For this review, take the finished solid that the model builds, in its own axes (mm). Face numbers are marked on the shaded views. A direction names the side the tool comes from. Give positions to 0.01 mm unless a question says otherwise; leave off trailing zeros. Loops run counter-clockwise (first coordinate to the right, second up) from the corner with the lowest first, then second, coordinate; pieces in that order, holes last.
```python
from build123d import *

# Parameters (mm, degrees)
SKETCH1_R           = 6.5
SKETCH1_R_2         = 7.5
BOSS_EXTRUDE1_DEPTH = 15
FILLET2_R           = 1.5
SKETCH4_R           = 3
CUT_EXTRUDE1_DEPTH  = 28


with BuildPart() as part:
    # Sketch1 → Boss-Extrude1 (new body)
    with BuildSketch(Plane.XY):
        with BuildLine():
            Line((-13.5, 0), (-13.5, -24))
            ThreePointArc((-13.5, -24), (-13.060660172, -25.060660172), (-12, -25.5))
            Line((-12, -25.5), (-9.5, -25.5))
            ThreePointArc((-9.5, -25.5), (-8.439339828, -25.939339828), (-8, -27))
            Line((-8, -27), (-8, -175.723012342))
            ThreePointArc((-8, -175.723012342), (0, -197.25), (8, -175.723012342))
            Line((8, -175.723012342), (8, -27))
            ThreePointArc((8, -27), (8.439339828, -25.939339828), (9.5, -25.5))
            Line((9.5, -25.5), (12, -25.5))
            ThreePointArc((12, -25.5), (13.060660172, -25.060660172), (13.5, -24))
            Line((13.5, -24), (13.5, 0))
            ThreePointArc((13.5, 0), (0, 13.5), (-13.5, 0))
        make_face()
        with Locations((0, -185)):
            Circle(SKETCH1_R, mode=Mode.SUBTRACT)
        Circle(SKETCH1_R_2, mode=Mode.SUBTRACT)
    extrude(amount=BOSS_EXTRUDE1_DEPTH)

    # Fillet2
    fillet2_edges = [part.edges().sort_by_distance(p)[0] for p in [
        (-13.060660172, -25.060660172, 15),
        (-10.75, -25.5, 15),
        (-8.439339828, -25.939339828, 15),
        (-8, -101.361506171, 15),
        (8, -101.361506171, 15),
        (8.439339828, -25.939339828, 15),
        (10.75, -25.5, 15),
        (13.060660172, -25.060660172, 15),
        (13.5, -12, 15),
        (0, 13.5, 15),
        (-13.5, -12, 15),
    ]]
    fillet(fillet2_edges, radius=FILLET2_R)

    # Sketch4 → Cut-Extrude1 (cut, through all)
    with BuildSketch(Plane(origin=(13.5, 0, 0), x_dir=(0, 0, -1), z_dir=(1, 0, 0))):
        with Locations((-6.75, -8)):
            Circle(SKETCH4_R)
    extrude(amount=-CUT_EXTRUDE1_DEPTH, mode=Mode.SUBTRACT)


solid = part.part
```
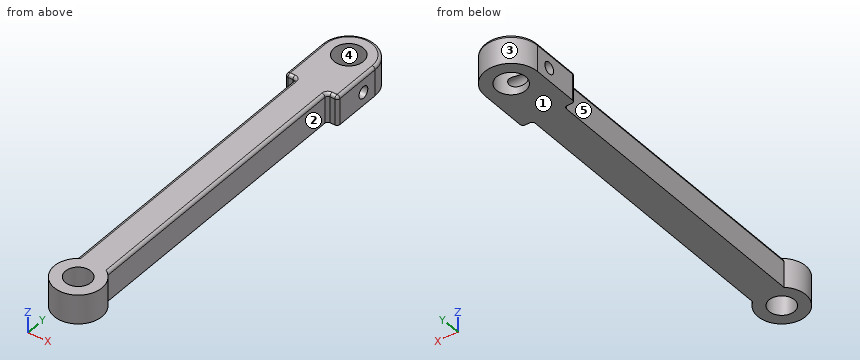
Item 1: Tool access review of the marked faces 4 and 5: name each direction out of +Z, -Z, +X, -X, +Y, -Y from which nothing blocks a thin tool from reaching the whole face with its end or side.
Answer:
face 4: +Z, -Z
face 5: +Z, -Z, -X
Item 2: Take a section at B-B on z = 6.25. Give the boundary of the cut face in (x, y), and give its area (3 significant figures).
Answer:
outline: (-13.5, -24) arc R1.5 ccw to (-12, -25.5) - (-9.5, -25.5) arc R1.5 cw to (-8, -27) - (-8, -175.72) arc R12.25 ccw (long way) to (8, -175.72) - (8, -27) arc R1.5 cw to (9.5, -25.5) - (12, -25.5) arc R1.5 ccw to (13.5, -24) - (13.5, -10.96) - (-13.5, -10.96) - close; (-13.5, -5.04) - (-5.55, -5.04) arc R7.5 cw (long way) to (5.55, -5.04) - (13.5, -5.04) - (13.5, 0) arc R13.5 ccw to (-13.5, 0) - close; hole circle Ø13 at (0, -185)
area: 3,370 mm2
Item 3: For L1, parallel to Y at x = 0, z = 6.75; L2, parallel to Y at x = -1, z = 6; L3, parallel to X at y = -50, z = 11.5, list the stretches that pass through material, from the lowest coordinate up.
Answer:
L1: y = -197.25 to -191.5, -178.5 to -11, 7.5 to 13.5
L2: y = -197.21 to -191.42, -178.58 to -10.9, 7.43 to 13.46
L3: x = -8 to 8
Item 4: Take a section at A-A on y = -185. Give the boundary of the cut face in (x, z), and give its area (4 significant figures).
Answer:
outline: (-12.25, 0) - (-6.5, 0) - (-6.5, 15) - (-12.25, 15) - close; (6.5, 0) - (12.25, 0) - (12.25, 15) - (6.5, 15) - close
area: 172.5 mm2
Item 5: Take a section at C-C on y = -112.5. Give the boundary of the cut face in (x, z).
Answer:
outline: (-8, 0) - (8, 0) - (8, 13.5) arc R1.5 ccw to (6.5, 15) - (-6.5, 15) arc R1.5 ccw to (-8, 13.5) - close
Item 6: The part is to be moulded in two halves that separate along Y. For the marked faces 1, 2 and 3, say which applies: released by +Y, released by -Y, zero draft, split by the parting line, or undercut.
Answer:
face 1: zero draft
face 2: undercut
face 3: released by +Y
Item 7: Clearance check with flat-ended pins moving along their axes: pin 1 Ø3 at (x, z) = (-10.5, 4) entering from -Y; pin 2 Ø1.5 at (x, z) = (-8.5, 5) entering from -Y; pin 3 Ø5 at (y, z) = (-125.5, 3.5) entering from +X. State where each tip first meets the part, or that it passes through.
Answer:
pin 1: stops at y = -193.31
pin 2: stops at y = -194.49
pin 3: stops at x = 8
Item 8: Take a section at D-D on x = -2. State how many separate pieces and enclosed holes the cut face has, and give its area (3 significant figures).
Answer:
separate pieces: 3
enclosed holes: 0
area: 2,730 mm2
